Geometry check sheet. Reference: the model listing, model coordinates, mm. Round coordinates to 2 decimals unless told otherwise and drop trailing zeros. Write each loop counter-clockwise with the first axis right and the second up, starting at its lowest first coordinate (ties: lowest second). Pieces come first, ordered by that corner, then holes. Notation, with made-up numbers: M 17,35 L 33,35 A27 ccw 33,73 Z; hole C 37.25,78.25 d3. An arc over 180 degrees is marked long. Use a Markdown table: item, result.
```python
from build123d import *

# Parameters (mm, degrees)
BOSS_EXTRUDE1_DEPTH = 9.525
FILLET1_R           = 0.396875


with BuildPart() as part:
    # Sketch1 → Boss-Extrude1 (new body)
    with BuildSketch(Plane(origin=(0, 0, 0), x_dir=(0, 0, -1), z_dir=(1, 0, 0))):
        with BuildLine():
            ThreePointArc((0.83712048, 0), (-0.050318999, 1.984375), (-0.937758477, 0))
            ThreePointArc((-0.937758477, 0), (-0.050318999, -1.984375), (0.83712048, 0))
        make_face()
        with BuildLine():
            ThreePointArc((0.54130732, 0.264583333), (-0.050318999, 1.5875), (-0.641945318, 0.264583333))
            ThreePointArc((-0.641945318, 0.264583333), (-0.540883477, 0), (-0.641945318, -0.264583333))
            ThreePointArc((-0.641945318, -0.264583333), (-0.050318999, -1.5875), (0.54130732, -0.264583333))
            ThreePointArc((0.54130732, -0.264583333), (0.44024548, 0), (0.54130732, 0.264583333))
        make_face(mode=Mode.SUBTRACT)
    extrude(amount=BOSS_EXTRUDE1_DEPTH)

    # Fillet1
    fillet1_edges = [part.edges().sort_by_distance(p)[0] for p in [
        (4.7625, 0, 0.937758477),
        (4.7625, 0, -0.83712048),
    ]]
    fillet(fillet1_edges, radius=FILLET1_R)


solid = part.part
```
Item 1: Mould release check, pull along Y, two halves, no side actions. Record for faces 1 (the face through (0, 0.03, 0.86)), 2 (the face through (4.696, -1.984, 0.085)): +Y half, -Y half, draft (parallel to the pull), parting line (faces both ways), or undercut.
Outcome:
| item | result |
|---|---|
| face 1 | draft |
| face 2 | undercut |
Item 2: Go/stop test with a flat-tipped pin: pin 1 (1 mm diameter, centred on x = 2.5, z = 1, fed in from +Y). Record where the tip stops, or that it passes through.
Outcome:
| item | result |
|---|---|
| pin 1 | stops at y = 1.9 |
Item 3: Material ranges on line 1 along Y through (x, z) = (3, 0); line 2 along Y through (x, z) = (3, -0.55); line 3 along Y through (x, z) = (3, 0.5), recorded low to high. Write a range as from..to.
Outcome:
| item | result |
|---|---|
| line 1 | y = -1.98..-1.59, 1.59..1.98 |
| line 2 | y = -1.82..-1.31, -0.27..0.27, 1.31..1.82 |
| line 3 | y = -1.9..-1.45, 1.45..1.9 |
Item 4: Cross-section at C-C, the plane z = 0.75. Record the cut outline in (x, y) (3 decimals), and give its area (3 significant figures).
Outcome:
| item | result |
|---|---|
| outline | M 0,-1.757 L 9.525,-1.757 L 9.525,-1.169 L 0,-1.169 Z; M 0,-0.419 L 9.525,-0.419 L 9.525,0.419 L 0,0.419 Z; M 0,1.169 L 9.525,1.169 L 9.525,1.757 L 0,1.757 Z |
| area | 19.2 mm2 |
Item 5: Cross-section at D-D, the plane y = 1.7. Record the cut outline in (x, z) (3 decimals), and give its area (3 significant figures).
Outcome:
| item | result |
|---|---|
| outline | M 0,-0.722 L 9.525,-0.722 L 9.525,0.823 L 0,0.823 Z |
| area | 14.7 mm2 |
Item 6: Cross-section at B-B, the plane y = 0.5. Record the cut outline in (x, z) (1 decimal), and give its area (3 significant figures).
Outcome:
| item | result |
|---|---|
| outline | M 0,-1.1 L 9.5,-1.1 L 9.5,-0.7 L 0,-0.7 Z; M 0,0.8 L 9.5,0.8 L 9.5,1.2 L 0,1.2 Z |
| area | 7.93 mm2 |
